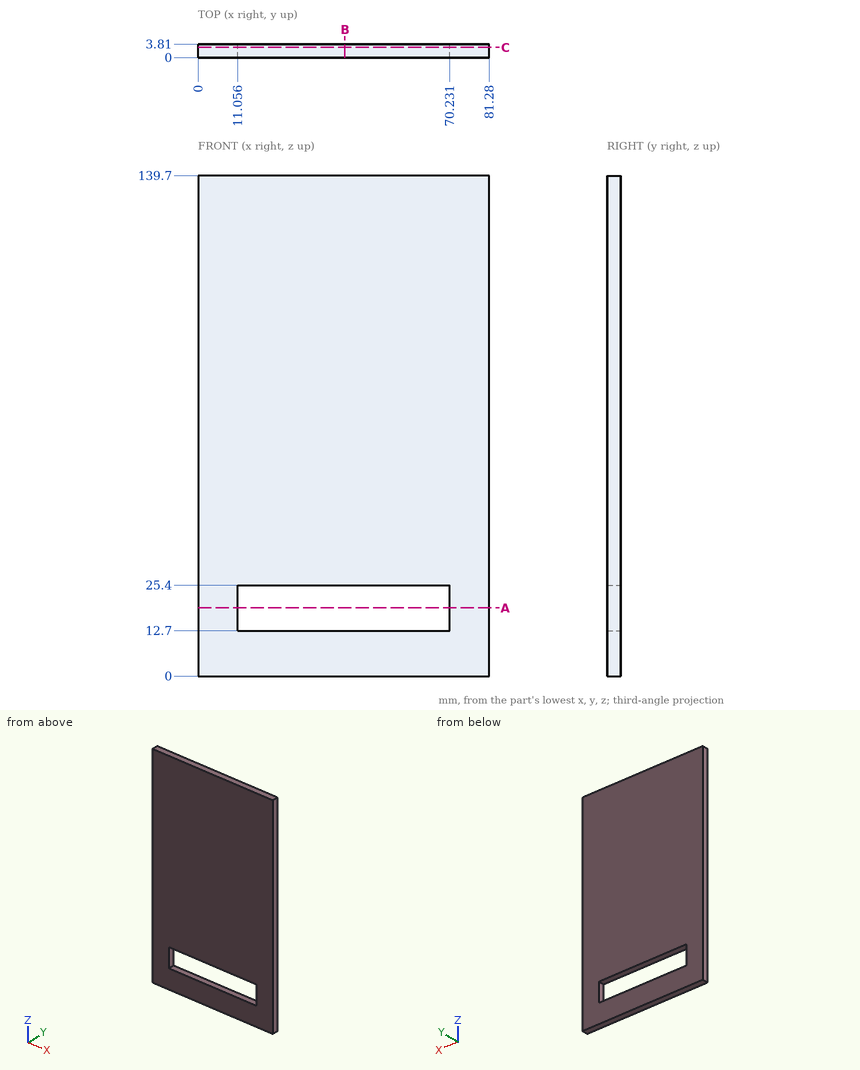
Part print with two shaded views. Sizes in mm from the minimum x, y, z corner. Round coordinates to 2 decimals unless told otherwise and drop trailing zeros. Order: outer loops, then holes, each group sorted by start corner. A loop starts at its lowest first (then second) coordinate and runs counter-clockwise, first axis right, second up. Notation, with made-up numbers: M 80.5,78.25 L 106.5,78.25 A7 cw 106.5,90.25 Z; hole C -31,69 d2. An arc over 180 degrees is marked long. Answer in a Markdown table with one row per item. Add a question column.
Q1. Cut at C-C on y = 2.9. Give the cut face in (x, z).
Q2. Cut at B-B on x = 41. Give the cut face in (y, z), and give its area (3 significant figures).
Q3. Wall check: L1, parallel to Z at x = 35.5, y = 1.85. Give the ranges that are in metal, low to high. Write a range as from..to.
Q4. Cut at A-A on z = 19. Give the cut face in (x, y).
Established:
| question | item | result |
|---|---|---|
| 1 | outline | M 0,0 L 81.28,0 L 81.28,139.7 L 0,139.7 Z; hole M 11.06,12.7 L 70.23,12.7 L 70.23,25.4 L 11.06,25.4 Z |
| 2 | outline | M 0,0 L 3.81,0 L 3.81,12.7 L 0,12.7 Z; M 0,25.4 L 3.81,25.4 L 3.81,139.7 L 0,139.7 Z |
| 2 | area | 484 mm2 |
| 3 | L1 | z = 0..12.7, 25.4..139.7 |
| 4 | outline | M 0,0 L 11.06,0 L 11.06,3.81 L 0,3.81 Z; M 70.23,0 L 81.28,0 L 81.28,3.81 L 70.23,3.81 Z |
